Design review of the part built by this model. Coordinates are the model's own, in mm. Coordinates: 2 decimals unless noted, no trailing zeros. Loops run counter-clockwise (first coordinate to the right, second up) from the corner with the lowest first, then second, coordinate; pieces in that order, holes last. Notation, with made-up numbers: M 89,-16.75 L 100,-16.75 A32 cw 100,9.25 Z; hole C -27.5,12.5 d11. An arc over 180 degrees is marked long. Write item = value, one per line. Start each with the question number.
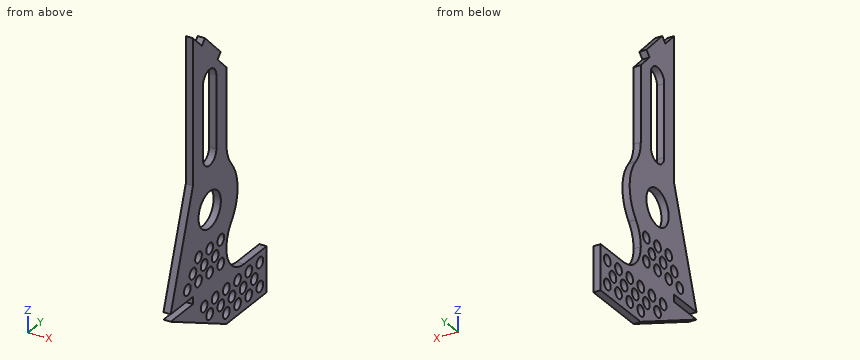
```python
from build123d import *

# Parameters (mm, degrees)
SKETCH2_R           = 10
SKETCH2_R_2         = 3
BOSS_EXTRUDE1_DEPTH = 4


with BuildPart() as part:
    # Sketch2 → Boss-Extrude1 (new body)
    with BuildSketch(Plane(origin=(0, 0, 0), x_dir=(0, 0, -1), z_dir=(1, 0, 0))):
        with BuildLine():
            Line((119, 9), (119, 44.995728753))
            Line((119, 44.995728753), (94, 44.995728753))
            Line((94, 44.995728753), (94, 24.715728753))
            ThreePointArc((94, 24.715728753), (89.39696962, 13.60303038), (78.284271247, 9))
            ThreePointArc((78.284271247, 9), (71.617604581, 10.143819168), (65.713484026, 13.444444444))
            ThreePointArc((65.713484026, 13.444444444), (50, 19), (34.286515974, 13.444444444))
            ThreePointArc((34.286515974, 13.444444444), (28.382395419, 10.143819168), (21.715728753, 9))
            Line((21.715728753, 9), (-20, 9))
            Line((-20, 9), (-27.928932188, 1.071067812))
            Line((-27.928932188, 1.071067812), (-30.757359313, 3.899494937))
            Line((-30.757359313, 3.899494937), (-44.899494937, -10.242640687))
            Line((-44.899494937, -10.242640687), (-42.071067812, -13.071067812))
            Line((-42.071067812, -13.071067812), (-50, -21))
            Line((-50, -21), (18.196601125, -21))
            Line((18.196601125, -21), (30, -21))
            Line((30, -21), (90, -41))
            Line((90, -41), (90, -21))
            Line((90, -21), (94, -21))
            Line((94, -21), (94, -41))
            Line((94, -41), (119, 9))
        make_face()
        with Locations((50, -6)):
            Circle(SKETCH2_R, mode=Mode.SUBTRACT)
        with Locations((106.5, -6)):
            Circle(SKETCH2_R_2, mode=Mode.SUBTRACT)
        with Locations((106.5, 4)):
            Circle(SKETCH2_R_2, mode=Mode.SUBTRACT)
        with Locations((113, 9)):
            Circle(SKETCH2_R_2, mode=Mode.SUBTRACT)
        with Locations((106.5, 14)):
            Circle(SKETCH2_R_2, mode=Mode.SUBTRACT)
        with Locations((113, 19)):
            Circle(SKETCH2_R_2, mode=Mode.SUBTRACT)
        with Locations((106.5, 24)):
            Circle(SKETCH2_R_2, mode=Mode.SUBTRACT)
        with Locations((113, 29)):
            Circle(SKETCH2_R_2, mode=Mode.SUBTRACT)
        with Locations((113, 39)):
            Circle(SKETCH2_R_2, mode=Mode.SUBTRACT)
        with Locations((106.5, 34)):
            Circle(SKETCH2_R_2, mode=Mode.SUBTRACT)
        with Locations((100, 39)):
            Circle(SKETCH2_R_2, mode=Mode.SUBTRACT)
        with Locations((100, 29)):
            Circle(SKETCH2_R_2, mode=Mode.SUBTRACT)
        with Locations((100, 19)):
            Circle(SKETCH2_R_2, mode=Mode.SUBTRACT)
        with Locations((100, 9)):
            Circle(SKETCH2_R_2, mode=Mode.SUBTRACT)
        with Locations((100, -1)):
            Circle(SKETCH2_R_2, mode=Mode.SUBTRACT)
        with Locations((100, -11)):
            Circle(SKETCH2_R_2, mode=Mode.SUBTRACT)
        with Locations((84, 4)):
            Circle(SKETCH2_R_2, mode=Mode.SUBTRACT)
        with Locations((71, 4)):
            Circle(SKETCH2_R_2, mode=Mode.SUBTRACT)
        with Locations((77.5, -1)):
            Circle(SKETCH2_R_2, mode=Mode.SUBTRACT)
        with Locations((84, -6)):
            Circle(SKETCH2_R_2, mode=Mode.SUBTRACT)
        with Locations((84, -16)):
            Circle(SKETCH2_R_2, mode=Mode.SUBTRACT)
        with Locations((77.5, -11)):
            Circle(SKETCH2_R_2, mode=Mode.SUBTRACT)
        with Locations((71, -6)):
            Circle(SKETCH2_R_2, mode=Mode.SUBTRACT)
        with Locations((71, -16)):
            Circle(SKETCH2_R_2, mode=Mode.SUBTRACT)
        with Locations((84, -26)):
            Circle(SKETCH2_R_2, mode=Mode.SUBTRACT)
        with Locations((77.5, -21)):
            Circle(SKETCH2_R_2, mode=Mode.SUBTRACT)
        with BuildLine():
            Line((20, 0), (-20, 0))
            ThreePointArc((-20, 0), (-26, -6), (-20, -12))
            Line((-20, -12), (20, -12))
            ThreePointArc((20, -12), (26, -6), (20, 0))
        make_face(mode=Mode.SUBTRACT)
    extrude(amount=BOSS_EXTRUDE1_DEPTH)


solid = part.part
```
(1) Take a section at B-B (z = -71). State the section outline as (x, y) points, plus the area to 3 significant figures.
(2) Take a section at D-D (x = 1.3). Give the number of separate pieces and of enclosed holes in the cut face, plus the area to 3 significant figures.
(3) Take a section at A-A (y = 34). State the section outline as (x, z) points, plus the area to 3 significant figures.
(4) Take a section at C-C (z = -45). State the section outline as (x, y) points.
(5) To check wall thickness, follow L1, parallel to Y at x = 1.25, z = -18; L2, parallel to Y at x = 2.4, z = -77.5; L3, parallel to Y at x = 2.15, z = -71. State the ranges of each line that lie inside material, in increasing order.
Results list:
q1.outline = M 0,-34.67 L 4,-34.67 L 4,-19 L 0,-19 Z; M 0,-13 L 4,-13 L 4,-9 L 0,-9 Z; M 0,-3 L 4,-3 L 4,1 L 0,1 Z; M 0,7 L 4,7 L 4,10.37 L 0,10.37 Z
q1.area = 108 mm^2
q2.separate_pieces = 1
q2.enclosed_holes = 27
q2.area = 4,810 mm^2
q3.outline = M 0,-119 L 4,-119 L 4,-109.5 L 0,-109.5 Z; M 0,-103.5 L 4,-103.5 L 4,-94 L 0,-94 Z
q3.area = 76.0 mm^2
q4.outline = M 0,-26 L 4,-26 L 4,-14.66 L 0,-14.66 Z; M 0,2.66 L 4,2.66 L 4,18.49 L 0,18.49 Z
q5.L1 = -21 to -12, 0 to 9
q5.L2 = -36.83 to -24, -18 to -14, -8 to -4, 2 to 9.02
q5.L3 = -34.67 to -19, -13 to -9, -3 to 1, 7 to 10.37
